from build123d import *

# Parameters (mm, degrees)
F0_R     = 30
F1_DEPTH = 30
F2_R     = 18
F3_DEPTH = 10
F5_D     = 22
F6_SIZE  = 2.54
F7_SIZE  = 2.54


with BuildPart() as f1:
    # F0 (on Front) → F1 (new body)
    with BuildSketch(Plane.XZ):
        Circle(F0_R)
    extrude(amount=F1_DEPTH)

    # F2 (on face) → F3 (join)
    with BuildSketch(Plane.XZ.offset(30)):
        Circle(F2_R)
    extrude(amount=F3_DEPTH)

    # F5 (through all)
    with Locations(Plane.XZ.offset(40)):
        with Locations((0, 0)):
            Hole(F5_D / 2)

    # F6
    f6_edges = [f1.edges().sort_by_distance(p)[0] for p in [
        (-30, -30, 0),
    ]]
    chamfer(f6_edges, length=F6_SIZE)

    # F7
    f7_edges = [f1.edges().sort_by_distance(p)[0] for p in [
        (-18, -40, 0),
    ]]
    chamfer(f7_edges, length=F7_SIZE)


solid = f1.part
CAD build for the part. Positions are in the model's coordinates, mm. A direction names the side the tool comes from. Round coordinates to 2 decimals unless told otherwise and drop trailing zeros. Write each loop counter-clockwise with the first axis right and the second up, starting at its lowest first coordinate (ties: lowest second). Pieces come first, ordered by that corner, then holes. Notation, with made-up numbers: M -35.5,28.25 L 14.5,28.25 A16 ccw 14.5,48.25 Z; hole C -37,-10 d1. An arc over 180 degrees is marked long. Use a Markdown table: item, result. Add a question column.
1. 3-axis set-ups, long thin cutter, end or side, ignore diameter. For faces 4 (the face through (18, -30, -6)), 5 (the face through (-29.97, -13.54, 1.32)): which of +Z, -Z, +X, -X, +Y, -Y reach the whole face in a straight line?
2. Slice it at B-B on z = 0. Give the cut face in (x, y), then the cut area to 3 significant figures.
3. Slice it at D-D on y = -35.5. Give the cut face in (x, z), then the cut area to 3 significant figures.
4. Slice it at A-A on x = 0. Give the cut face in (y, z).
5. Slice it at C-C on y = -19. Give the cut face in (x, z), then the cut area to 3 significant figures.
6. Flat gauge pins, fed straight in: P1, Ø8, axis at y = -21.5, z = -5.5, coming from the -X side; P2, Ø12, axis at x = -16, y = -17, coming from the -Z side; P3, Ø1, axis at y = -21.5, z = -4, coming from the -X side; P4, Ø4, axis at y = -6, z = 1, coming from the +X side. Where does each tip first touch, or does it go through?
7. Drill centre lines: probe 1 along Z at (x, y) = (0, -11); probe 2 along X at (y, z) = (-12, 10); probe 3 along Y at (x, z) = (-5, 23.5). Where is each one in solid material? Low to high.
8. Pull direction X, two halves, no side cores. Call faces 1 (the face through (13, 0, 0)), 2 (the face through (2.38, -19.72, -10.74)), 3 (the face through (-2.343, -33.678, 17.847)): released by +X, released by -X, zero draft, split by the parting line, or undercut.
Reply:
| question | item | result |
|---|---|---|
| 1 | face 4 | -Y |
| 1 | face 5 | +Y, -Y |
| 2 | outline | M -30,-27.46 L -27.46,-30 L -18,-30 L -18,-37.46 L -15.46,-40 L -11,-40 L -11,0 L -30,0 Z; M 11,-40 L 15.46,-40 L 18,-37.46 L 18,-30 L 27.46,-30 L 30,-27.46 L 30,0 L 11,0 Z |
| 2 | area | 1,270 mm^2 |
| 3 | outline | C 0,0 d36; hole C 0,0 d22 |
| 3 | area | 638 mm^2 |
| 4 | outline | M -40,-15.46 L -37.46,-18 L -30,-18 L -30,-27.46 L -27.46,-30 L 0,-30 L 0,-11 L -40,-11 Z; M -40,11 L 0,11 L 0,30 L -27.46,30 L -30,27.46 L -30,18 L -37.46,18 L -40,15.46 Z |
| 5 | outline | C 0,0 d60; hole C 0,0 d22 |
| 5 | area | 2,450 mm^2 |
| 6 | P1 | stops at x = -29.96 |
| 6 | P2 | stops at z = -28.28 |
| 6 | P3 | stops at x = -29.8 |
| 6 | P4 | stops at x = 30 |
| 7 | probe 1 | z = -30 to -11, 11 to 30 |
| 7 | probe 2 | x = -28.28 to -4.58, 4.58 to 28.28 |
| 7 | probe 3 | y = -30 to 0 |
| 8 | face 1 | zero draft |
| 8 | face 2 | undercut |
| 8 | face 3 | split by the parting line |
